For this review, take the finished solid that the model builds, in its own axes (mm). Coordinates: 2 decimals unless noted, no trailing zeros. Loops run counter-clockwise (first coordinate to the right, second up) from the corner with the lowest first, then second, coordinate; pieces in that order, holes last. Notation, with made-up numbers: M 20.5,83.25 L 63.5,83.25 A22 ccw 63.5,121.25 Z; hole C 66,-36 d1. An arc over 180 degrees is marked long. Use one line per item in the form item = value.
```python
from build123d import *

# Parameters (mm, degrees)
SKETCH1_W           = 3.175
SKETCH1_H           = 3.175
BOSS_EXTRUDE1_DEPTH = 31.75
SKETCH2_OUTSIDE_W   = 11.588
SKETCH2_OUTSIDE_H   = 11.589
SKETCH2_OUTSIDE_R   = 2.032
CUT_EXTRUDE1_DEPTH  = 32.75


with BuildPart() as part:
    # Sketch1 → Boss-Extrude1 (new body)
    with BuildSketch(Plane.XY):
        Rectangle(SKETCH1_W, SKETCH1_H)
    extrude(amount=BOSS_EXTRUDE1_DEPTH)

    # Sketch2 outside → Cut-Extrude1 (cut, through all)
    with BuildSketch(Plane(origin=(0, 0, 0), x_dir=(-1, 0, 0), z_dir=(0, 0, -1))):
        with Locations((0, -0.0005)):
            Rectangle(SKETCH2_OUTSIDE_W, SKETCH2_OUTSIDE_H)
        Circle(SKETCH2_OUTSIDE_R, mode=Mode.SUBTRACT)
    extrude(amount=-CUT_EXTRUDE1_DEPTH, mode=Mode.SUBTRACT)

    # Sketch3 → Cut-Revolve1 (revolve, cut)
    with BuildSketch(Plane(origin=(0, 0, 0), x_dir=(1, 0, 0), z_dir=(0, 1, 0))):
        with BuildLine():
            Line((-5.053685963, -4.40273269), (-5.053685963, 5.740530545))
            Line((-5.053685963, 5.740530545), (0, 5.740530545))
            Line((0, 5.740530545), (0, 0.160877736))
            ThreePointArc((0, 0.160877736), (-3.404639553, -1.148866368), (-5.053685963, -4.40273269))
        make_face()
    revolve(axis=Axis((0, 0, 31.75), (0, 0, -1)), mode=Mode.SUBTRACT)

    # Mirror1: part across plane


with BuildPart() as part_1:
    add(part.part)
    add(part.part.mirror(Plane(origin=(0, 0, 31.75), x_dir=(1, 0, 0), z_dir=(0, 0, -1))))


solid = part_1.part
```
1. Consider section A-A on z = 17.5. Write out the cut boundary in (x, y).
Computed values:
outline = M -1.59,-1.27 A2.03 ccw -1.27,-1.59 L 1.27,-1.59 A2.03 ccw 1.59,-1.27 L 1.59,1.27 A2.03 ccw 1.27,1.59 L -1.27,1.59 A2.03 ccw -1.59,1.27 Z
2. Wall thickness on line 1 along Z through (x, y) = (-1.35, 1); line 2 along Z through (x, y) = (-1.3, 0.6); line 3 along X through (y, z) = (1.35, 42): over which ranges is each line inside the solid? List them lowest first. Write a range as from..to.
Computed values:
line_1 = 0.12..63.38
line_2 = 0.05..63.45
line_3 = -1.52..1.52
3. For pin 1 Ø1 at (x, y) = (1, -0.5) entering from -Z, flat-tipped, find the tip position at first contact; note if it passes through.
Computed values:
pin_1 = 0
4. Draft analysis for pull direction X (two halves, no side actions). For faces 1 (the face through (1.588, 0, 32)), 2 (the face through (-1.588, 0, 32)), 3 (the face through (0, -1.588, 32)), state which applies: +X half, -X half, draft (parallel to the pull), parting line (faces both ways), or undercut.
Computed values:
face_1 = +X half
face_2 = -X half
face_3 = draft
